```python
from build123d import *

# Parameters (mm, degrees)
F1_DEPTH = 10
F2_D     = 6
F4_D     = 3.3
F4_DEPTH = 15.5
F4_TIP   = 0.9914200214
F6_D     = 3.3
F6_DEPTH = 20
F6_TIP   = 0.9914200214
F9_D     = 7
F9_DEPTH = 7
F9_TIP   = 2.1030121666


with BuildPart() as f1:
    # F0 (on Top) → F1 (new body)
    with BuildSketch(Plane.XY):
        Polygon((-20, 10.239787288), (-20, -5), (20, -5), (20, 10.239787288), (12, 10.239787288), (10.6523660943, 10.239787288), (-9.4155045226, 10.239787288), (-12, 10.239787288), align=None)
    extrude(amount=F1_DEPTH)

    # F2 (through all)
    with Locations(Plane(origin=(0, 0, 0), x_dir=(1, 0, 0), z_dir=(0, 0, -1))):
        with Locations((0, -5.239787288)):
            Hole(F2_D / 2)

    # F4
    with Locations(Plane.XZ.offset(5)):
        with Locations((-10, 5), (10, 5)):
            Hole(F4_D / 2, depth=F4_DEPTH)
            with Locations((0, 0, -(F4_DEPTH + F4_TIP / 2))):  # 118° drill point
                Cone(0, F4_D / 2, F4_TIP, mode=Mode.SUBTRACT)

    # F6
    with Locations(Plane(origin=(-20, 0, 0), x_dir=(0, -1, 0), z_dir=(-1, 0, 0))):
        with Locations((-5.239787288, 5)):
            Hole(F6_D / 2, depth=F6_DEPTH)
            with Locations((0, 0, -(F6_DEPTH + F6_TIP / 2))):  # 118° drill point
                Cone(0, F6_D / 2, F6_TIP, mode=Mode.SUBTRACT)

    # F9
    with Locations(Plane.XY.offset(10)):
        with Locations((0, 5.2691735327)):
            Hole(F9_D / 2, depth=F9_DEPTH)
            with Locations((0, 0, -(F9_DEPTH + F9_TIP / 2))):  # 118° drill point
                Cone(0, F9_D / 2, F9_TIP, mode=Mode.SUBTRACT)


solid = f1.part
```
Read the model definition and answer for the solid it produces. Units are mm, in the model's axes. A direction names the side the tool comes from. Give positions to 0.01 mm unless a question says otherwise; leave off trailing zeros. Loops run counter-clockwise (first coordinate to the right, second up) from the corner with the lowest first, then second, coordinate; pieces in that order, holes last.
Item 1: Find the intervals of material crossed by line 1 along Y through (x, z) = (0, 0.65); line 2 along X through (y, z) = (-2.5, 5.75); line 3 along Y through (x, z) = (-12, 5), in increasing order.
Item 2: The mould has two halves that part along Y. Classify faces 4 (the flat face through (0, 10.24, 5)), 5 (the cylindrical face through (-6.487, 5.025, 6.636)), 6 (the cylindrical face through (-11.524, 0.192, 4.368)): released by +Y, released by -Y, zero draft, split by the parting line, or undercut.
Item 3: The part is cut by section D-D (z = 2.25). Write down the section's boundary in (x, y).
Item 4: The part is cut by section B-B (z = 5.5). Write down the section's boundary in (x, y).
Item 5: This flat-tipped pin is pushed along its axis until it touches: pin 1 Ø6.5 at (x, y) = (0, 5.27) entering from +Z. Where does it stop, or does it pass through?
Item 6: The part is cut by section C-C (y = 0.75). Write down the section's boundary in (x, z).
Item 7: The part is cut by section A-A (x = 0). Write down the section's boundary in (y, z).
Item 8: For faces 1 (the cylindrical face through (-14.93, 6.764, 4.368)), 2 (the flat face through (-20, 3, 5)), 3 (the cylindrical face through (3.497, 5.423, 6.451)), determine the directions among +Z, -Z, +X, -X, +Y, -Y from which every point of the face is accessible in a straight line to the end or side of a thin tool.
Taken from the geometry:
1. line 1: y = -5 to 2.24, 8.24 to 10.24
1. line 2: x = -20 to -11.47, -8.53 to 8.53, 11.47 to 20
1. line 3: y = -5 to 3.59, 6.89 to 10.24
2. face 4: released by +Y
2. face 5: undercut
2. face 6: zero draft
3. outline: (-20, -5) - (20, -5) - (20, 10.24) - (-20, 10.24) - close; hole circle Ø6 at (0, 5.24)
4. outline: (-20, -5) - (-11.57, -5) - (-11.57, 3.67) - (-20, 3.67) - close; (-20, 6.81) - (-11.57, 6.81) - (-11.57, 10.24) - (-20, 10.24) - close; (-8.43, -5) - (8.43, -5) - (8.43, 10.24) - (-8.43, 10.24) - (-8.43, 6.81) - (-3.14, 6.81) arc R3.5 cw (long way) to (-3.11, 3.67) - (-8.43, 3.67) - close; (11.57, -5) - (20, -5) - (20, 10.24) - (11.57, 10.24) - close
5. pin 1: stops at z = 2.85
6. outline: (-20, 0) - (20, 0) - (20, 10) - (-20, 10) - close; hole circle Ø3.3 at (-10, 5); hole circle Ø3.3 at (10, 5)
7. outline: (-5, 0) - (2.24, 0) - (2.24, 2.72) - (1.77, 3) - (1.77, 10) - (-5, 10) - close; (8.24, 0) - (10.24, 0) - (10.24, 10) - (8.77, 10) - (8.77, 3) - (8.24, 2.68) - close
8. face 1: -X
8. face 2: +Z, -Z, -X, +Y, -Y
8. face 3: +Z
